```python
from build123d import *

# Parameters (mm, degrees)
F0_W     = 204
F0_H     = 80
F1_DEPTH = 70
F3_DEPTH = 69
F5_DEPTH = 2
F7_DEPTH = 14
F8_R     = 5
F9_R     = 0.49999


# Not quite as in the source:
# - a fillet or chamfer is up to 0.001 mm smaller than in the source, because OpenCascade refuses the exact size


with BuildPart() as f1:
    # F0 (on Top) → F1 (new body)
    with BuildSketch(Plane.XY):
        Rectangle(F0_W, F0_H)
    extrude(amount=F1_DEPTH)

    # F2 (on face) → F3 (cut)
    with BuildSketch(Plane.XY.offset(70)):
        Polygon((-70.4128742218, 39), (-101, 39), (-101, 20.586034283), (-101, -39), (-57.7337481081, -39), (100, -39), (100, -8.4424866363), (100, 39), align=None)
    extrude(amount=-F3_DEPTH, mode=Mode.SUBTRACT)

    # F4 (on face) → F5 (cut)
    with BuildSketch(Plane.YZ.offset(102)):
        Polygon((38, 2), (38, 70), (-38, 70), (-38, 42.2970801592), (-38, 2), align=None)
    extrude(amount=-F5_DEPTH, mode=Mode.SUBTRACT)

    # F6 (on face) → F7 (join)
    with BuildSketch(Plane(origin=(100, 0, 0), x_dir=(0, -1, 0), z_dir=(-1, 0, 0))):
        Polygon((39, 1), (39, 70), (38, 70), (38, 2), (-38, 2), (-38, 70), (-39, 70), (-39, 1), align=None)
    extrude(amount=-F7_DEPTH)

    # F8
    f8_edges = [f1.edges().sort_by_distance(p)[0] for p in [
        (-0.5, 39, 1),
        (-101, 0, 1),
        (-0.5, -39, 1),
        (0, 40, 0),
        (-102, 0, 0),
        (0, -40, 0),
        (-102, -40, 35),
        (-102, 40, 35),
        (-101, 39, 35.5),
        (-101, -39, 35.5),
        (108, 39, 1),
        (108, -39, 1),
        (107, -38, 2),
        (107, 38, 2),
    ]]
    fillet(f8_edges, radius=F8_R)

    # F9 (radius 0.5 in the source; OpenCascade refuses exactly that, so slightly less here)
    f9_edges = [f1.edges().sort_by_distance(p)[0] for p in [
        (2.5, 40, 70),
        (-100.535534, 38.535534, 70),
        (102, 39.5, 70),
        (-102, 0, 70),
        (108, 39, 70),
        (-100.535534, -38.535534, 70),
        (114, 38.5, 70),
        (2.5, -40, 70),
        (107, 38, 70),
        (102, -39.5, 70),
        (100, 38.5, 70),
        (108, -39, 70),
        (2, 39, 70),
        (114, -38.5, 70),
        (-99.535534, 37.535534, 70),
        (107, -38, 70),
        (-101, 0, 70),
        (100, -38.5, 70),
        (-99.535534, -37.535534, 70),
        (2, -39, 70),
        (114, -39, 38),
        (114, -37.535534, 2.464466),
        (114, 0, 1),
        (114, -38, 38.5),
        (114, 37.535534, 2.464466),
        (114, -36.535534, 3.464466),
        (114, 39, 38),
        (114, 0, 2),
        (114, 36.535534, 3.464466),
        (114, 38, 38.5),
    ]]
    fillet(f9_edges, radius=F9_R)


solid = f1.part
```
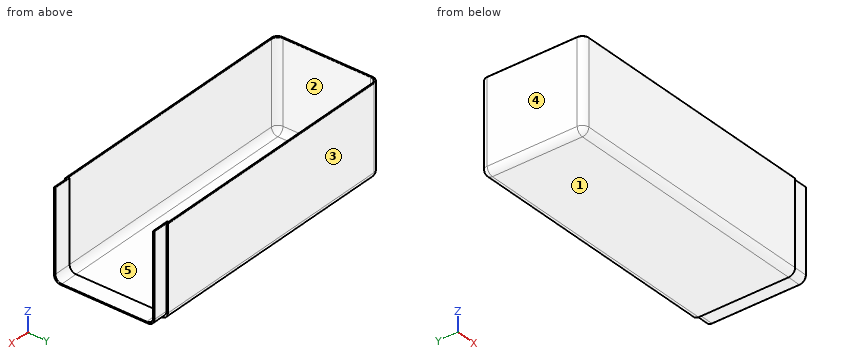
Check sheet for the modelled part. Datum: model origin and axes. Units: mm. Face numbers are marked on the shaded views. A direction names the side the tool comes from. Coordinates: 2 decimals unless noted, no trailing zeros. Write each question's results on one line, items separated by ' | '. Start each with the question number.
1. Access from +Z, -Z, +X, -X, +Y, -Y to the whole of each face (thin tool, end or side, straight path). Record for the marked faces 4 and 5.
2. Mould release check, pull along Y, two halves, no side actions. Record for the marked faces 1, 2 and 3: +Y half, -Y half, draft (parallel to the pull), parting line (faces both ways), or undercut.
3. Go/stop test with flat-tipped pins: P1, Ø4, axis at x = 105, y = -6.5, coming from the +Z side; P2, Ø12, axis at y = 3, z = 15, coming from the +X side; P3, Ø4, axis at x = 109.5, z = 44, coming from the -Y side. Record where each tip stops, or that it passes through.
4. Material ranges on probe 1 along Y at (x, z) = (82.5, 8); probe 2 along Y at (x, z) = (101, 22.5); probe 3 along X at (y, z) = (21, 24), recorded low to high.
Checks:
1) face 4: +Z, -Z, -X, +Y, -Y | face 5: +Z
2) face 1: draft | face 2: undercut | face 3: +Y half
3) P1: stops at z = 2 | P2: stops at x = -101 | P3: stops at y = -39
4) probe 1: y = -40 to -39, 39 to 40 | probe 2: y = -40 to -38, 38 to 40 | probe 3: x = -102 to -101
